from build123d import *
from OCP.BRepFilletAPI import BRepFilletAPI_MakeChamfer

# Parameters (mm, degrees)
SKETCH1_W           = 1.85
SKETCH1_H           = 38.85
SKETCH1_H_2         = 6.15
SKETCH1_W_2         = 44.85
SKETCH1_H_3         = 1.85
SKETCH1_W_3         = 0.15
BOSS_EXTRUDE1_DEPTH = 3
SKETCH1_4_W         = 120
SKETCH1_4_H         = 30
SKETCH1_4_W_2       = 30
SKETCH1_4_H_2       = 120
BOSS_EXTRUDE3_DEPTH = 4
BOSS_EXTRUDE9_DEPTH = 3
CHAMFER1_SIZE       = 2.5
CHAMFER1_SIZE2      = 9.330127019
SKETCH4_W           = 8.5
SKETCH4_H           = 30
SKETCH4_W_2         = 30
SKETCH4_H_2         = 8.5
CUT_EXTRUDE1_DEPTH  = 1.5
BOSS_EXTRUDE7_DEPTH = 4.7625
SKETCH10_R          = 14.258178215
CUT_EXTRUDE2_DEPTH  = 91.287114527
FILLET1_R           = 1.75
BOSS_EXTRUDE8_DEPTH = 4.7625
CUT_EXTRUDE3_DEPTH  = 97.69049149


with BuildPart() as part:
    # Sketch1 → Boss-Extrude1 (new body)
    with BuildSketch(Plane(origin=(0, 0, 0), x_dir=(-1, 0, 0), z_dir=(0, 0, -1))):
        with Locations((14.075, 40.575)):
            Rectangle(SKETCH1_W, SKETCH1_H)
        with Locations((14.075, 18.075)):
            Rectangle(SKETCH1_W, SKETCH1_H_2)
        with Locations((37.575, 14.075)):
            Rectangle(SKETCH1_W_2, SKETCH1_H_3)
        with Locations((14.075, 14.075)):
            Rectangle(SKETCH1_W, SKETCH1_H_3)
        with Locations((14.075, -14.075)):
            Rectangle(SKETCH1_W, SKETCH1_H_3)
        with Locations((14.075, -18.075)):
            Rectangle(SKETCH1_W, SKETCH1_H_2)
        with Locations((37.575, -14.075)):
            Rectangle(SKETCH1_W_2, SKETCH1_H_3)
        with Locations((14.075, -40.575)):
            Rectangle(SKETCH1_W, SKETCH1_H)
        with Locations((-14.075, -14.075)):
            Rectangle(SKETCH1_W, SKETCH1_H_3)
        with Locations((-14.075, -18.075)):
            Rectangle(SKETCH1_W, SKETCH1_H_2)
        with Locations((-37.575, -14.075)):
            Rectangle(SKETCH1_W_2, SKETCH1_H_3)
        with Locations((-15.075, -14.075)):
            Rectangle(SKETCH1_W_3, SKETCH1_H_3)
        with Locations((15.075, -14.075)):
            Rectangle(SKETCH1_W_3, SKETCH1_H_3)
        with Locations((15.075, 14.075)):
            Rectangle(SKETCH1_W_3, SKETCH1_H_3)
        with Locations((-37.575, 14.075)):
            Rectangle(SKETCH1_W_2, SKETCH1_H_3)
        with Locations((-15.075, 14.075)):
            Rectangle(SKETCH1_W_3, SKETCH1_H_3)
        with Locations((-14.075, 18.075)):
            Rectangle(SKETCH1_W, SKETCH1_H_2)
        with Locations((-14.075, 14.075)):
            Rectangle(SKETCH1_W, SKETCH1_H_3)
        with Locations((-14.075, 40.575)):
            Rectangle(SKETCH1_W, SKETCH1_H)
        with Locations((-14.075, -40.575)):
            Rectangle(SKETCH1_W, SKETCH1_H)
    extrude(amount=-BOSS_EXTRUDE1_DEPTH)

    # Sketch1<4> → Boss-Extrude3 (add)
    with BuildSketch(Plane(origin=(0, 0, 0), x_dir=(-1, 0, 0), z_dir=(0, 0, -1))):
        Rectangle(SKETCH1_4_W, SKETCH1_4_H)
        Rectangle(SKETCH1_4_W_2, SKETCH1_4_H_2)
    extrude(amount=BOSS_EXTRUDE3_DEPTH)

    # Sketch13 → Boss-Extrude9 (add)
    with BuildSketch(Plane.XY):
        Polygon((-12.2, 12.2), (-60, 12.2), (-60, 13.15), (-13.15, 13.15), (-13.15, 60), (-12.2, 60), align=None)
        Polygon((-60, -12.2), (-12.2, -12.2), (-12.2, -60), (-13.15, -60), (-13.15, -13.15), (-60, -13.15), align=None)
        Polygon((12.2, -60), (12.2, -12.2), (60, -12.2), (60, -13.15), (13.15, -13.15), (13.15, -60), align=None)
        Polygon((60, 12.2), (12.2, 12.2), (12.2, 60), (13.15, 60), (13.15, 13.15), (60, 13.15), align=None)
    extrude(amount=BOSS_EXTRUDE9_DEPTH)

    # Chamfer1: one chamfer whose edges measure the first distance from different faces: ONE call of the kernel's chamfer builder (chamfer() names one face for all edges)
    chamfer1_edges_1 = [part.edges().sort_by_distance(p)[0] for p in [
        (60, 0, -4),
    ]]
    chamfer1_side_1 = [part.faces().sort_by_distance(p)[0] for p in [
        (60, 0, -1.570175439),
    ]]
    chamfer1_edges_2 = [part.edges().sort_by_distance(p)[0] for p in [
        (0, 60, -4),
    ]]
    chamfer1_side_2 = [part.faces().sort_by_distance(p)[0] for p in [
        (0, 60, -1.570175439),
    ]]
    chamfer1_edges_3 = [part.edges().sort_by_distance(p)[0] for p in [
        (0, -60, -4),
    ]]
    chamfer1_side_3 = [part.faces().sort_by_distance(p)[0] for p in [
        (0, -60, -1.570175439),
    ]]
    chamfer1_edges_4 = [part.edges().sort_by_distance(p)[0] for p in [
        (-60, 0, -4),
    ]]
    chamfer1_side_4 = [part.faces().sort_by_distance(p)[0] for p in [
        (-60, 0, -1.570175439),
    ]]
    chamfer1 = BRepFilletAPI_MakeChamfer(part.part.solid().wrapped)
    for e in chamfer1_edges_1:
        chamfer1.Add(CHAMFER1_SIZE, CHAMFER1_SIZE2, e.wrapped, chamfer1_side_1[0].wrapped)  # the first distance lies on this face
    for e in chamfer1_edges_2:
        chamfer1.Add(CHAMFER1_SIZE, CHAMFER1_SIZE2, e.wrapped, chamfer1_side_2[0].wrapped)  # the first distance lies on this face
    for e in chamfer1_edges_3:
        chamfer1.Add(CHAMFER1_SIZE, CHAMFER1_SIZE2, e.wrapped, chamfer1_side_3[0].wrapped)  # the first distance lies on this face
    for e in chamfer1_edges_4:
        chamfer1.Add(CHAMFER1_SIZE, CHAMFER1_SIZE2, e.wrapped, chamfer1_side_4[0].wrapped)  # the first distance lies on this face
    add(Compound.cast(chamfer1.Shape()), mode=Mode.REPLACE)

    # Sketch4 → Cut-Extrude1 (cut)
    with BuildSketch(Plane(origin=(0, 0, -4), x_dir=(-1, 0, 0), z_dir=(0, 0, -1))):
        with Locations((-41.419872981, 0)):
            Rectangle(SKETCH4_W, SKETCH4_H)
        with Locations((-29.919872981, 0)):
            Rectangle(SKETCH4_W, SKETCH4_H)
        with Locations((0, 41.419872981)):
            Rectangle(SKETCH4_W_2, SKETCH4_H_2)
        with Locations((0, 29.919872981)):
            Rectangle(SKETCH4_W_2, SKETCH4_H_2)
        with Locations((29.919872981, 0)):
            Rectangle(SKETCH4_W, SKETCH4_H)
        with Locations((41.419872981, 0)):
            Rectangle(SKETCH4_W, SKETCH4_H)
        with Locations((0, -29.919872981)):
            Rectangle(SKETCH4_W_2, SKETCH4_H_2)
        with Locations((0, -41.419872981)):
            Rectangle(SKETCH4_W_2, SKETCH4_H_2)
    extrude(amount=-CUT_EXTRUDE1_DEPTH, mode=Mode.SUBTRACT)

    # Sketch9 → Boss-Extrude7 (add)
    with BuildSketch(Plane(origin=(-2.248627702, 2.248627702, 3.180039793), x_dir=(-0.86602540378444, -0.28867513459481, -0.40824829046386224), z_dir=(0.4999999999999977, -0.49999999999999806, -0.7071067811865507))):
        with BuildLine():
            Line((26.502649854, 26.860285477), (21.488288715, 19.768907948))
            Line((21.488288715, 19.768907948), (7.054531985, -0.643506575))
            Line((7.054531985, -0.643506575), (-2.958214479, 6.436574348))
            Line((-2.958214479, 6.436574348), (11.475542251, 26.848988872))
            Line((11.475542251, 26.848988872), (16.48990339, 33.940366401))
            ThreePointArc((16.48990339, 33.940366401), (25.036317083, 35.406699171), (26.502649854, 26.860285477))
        make_face()
        with BuildLine():
            ThreePointArc((19.161917241, 33.60764173), (16.307451178, 27.650713492), (22.309959452, 24.893384176))
            ThreePointArc((22.309959452, 24.893384176), (25.022858564, 30.799171082), (19.161917241, 33.60764173))
        make_face(mode=Mode.SUBTRACT)
    extrude(amount=BOSS_EXTRUDE7_DEPTH)

    # Sketch10 → Cut-Extrude2 (cut, through all)
    with BuildSketch(Plane.XY):
        Circle(SKETCH10_R)
    extrude(amount=CUT_EXTRUDE2_DEPTH, mode=Mode.SUBTRACT)

    # Fillet1
    fillet1_edges = [part.edges().sort_by_distance(p)[0] for p in [
        (-2.56318253, 2.56318253, -4),
        (-7.32568253, 7.32568253, -4),
        (-9.280078929, 0.60878613, -4),
        (-0.60878613, 9.280078929, -4),
    ]]
    fillet(fillet1_edges, radius=FILLET1_R)

    # Sketch11 → Boss-Extrude8 (add)
    with BuildSketch(Plane(origin=(-2.248627702, 2.248627702, 3.180039793), x_dir=(0.86602540378444, 0.28867513459481003, 0.4082482904638624), z_dir=(-0.4999999999999978, 0.4999999999999982, 0.7071067811865503))):
        with BuildLine():
            ThreePointArc((-26.502649854, 26.860285477), (-25.036317083, 35.406699171), (-16.48990339, 33.940366401))
            Line((-16.48990339, 33.940366401), (-7.126405249, 20.698380338))
            ThreePointArc((-7.126405249, 20.698380338), (-10.454022038, 27.858169656), (-11.039574704, 35.731716801))
            ThreePointArc((-11.039574704, 35.731716801), (-12.744347828, 41.802023869), (-18.161788795, 45.027890059))
            ThreePointArc((-18.161788795, 45.027890059), (-29.902759178, 42.288887582), (-36.398772273, 32.132395373))
            ThreePointArc((-36.398772273, 32.132395373), (-35.163210117, 25.949494318), (-30.008327436, 22.318783113))
            ThreePointArc((-30.008327436, 22.318783113), (-22.780260221, 19.142203051), (-17.139151713, 13.618299415))
            Line((-17.139151713, 13.618299415), (-26.502649854, 26.860285477))
        make_face()
    extrude(amount=-BOSS_EXTRUDE8_DEPTH)

    # Sketch12 → Cut-Extrude3 (cut, through all)
    with BuildSketch(Plane(origin=(-2.248627702, 2.248627702, 3.180039793), x_dir=(0.86602540378444, 0.28867513459481003, 0.4082482904638624), z_dir=(-0.4999999999999978, 0.4999999999999982, 0.7071067811865503))):
        Polygon((-25.756076527, 43.091629588), (-27.225983794, 42.459670234), (-25.971939452, 39.542823), (-24.502032185, 40.174782353), align=None)
        Polygon((-28.527874077, 41.730147071), (-26.694786972, 39.137770427), (-28.001181502, 38.214009996), (-29.834268606, 40.80638664), align=None)
        Polygon((-22.761781271, 43.84707133), (-24.330959276, 43.53453271), (-23.710765452, 40.420695106), (-22.141587447, 40.733233726), align=None)
        Polygon((-19.675853381, 43.963455868), (-21.275721515, 43.983997418), (-21.316483655, 40.809259091), (-19.716615522, 40.78871754), align=None)
        Polygon((-16.633162714, 43.435696639), (-18.193799062, 43.788420596), (-18.893735665, 40.691532844), (-17.333099317, 40.338808886), align=None)
        Polygon((-13.766689451, 42.286859254), (-15.219886716, 42.956349889), (-16.548407194, 40.072661566), (-15.095209929, 39.403170932), align=None)
        Polygon((-30.956033068, 39.822127099), (-32.04181915, 38.646938354), (-29.709803985, 36.492331599), (-28.624017903, 37.667520343), align=None)
        Polygon((-32.934431301, 37.450959299), (-33.752154873, 36.075703628), (-31.023131901, 34.453033416), (-30.205408329, 35.828289087), align=None)
        Polygon((-34.376603279, 34.720275083), (-34.890525897, 33.205057758), (-31.883766517, 32.185242563), (-31.3698439, 33.700459888), align=None)
        Polygon((-35.219519168, 31.749418455), (-35.407179947, 30.160461743), (-32.254093972, 29.788072384), (-32.066433193, 31.377029095), align=None)
        Polygon((-35.426339496, 28.668230104), (-35.279536761, 27.074979039), (-32.117929178, 27.366290716), (-32.264731914, 28.959541782), align=None)
    extrude(amount=-CUT_EXTRUDE3_DEPTH, mode=Mode.SUBTRACT)


solid = part.part
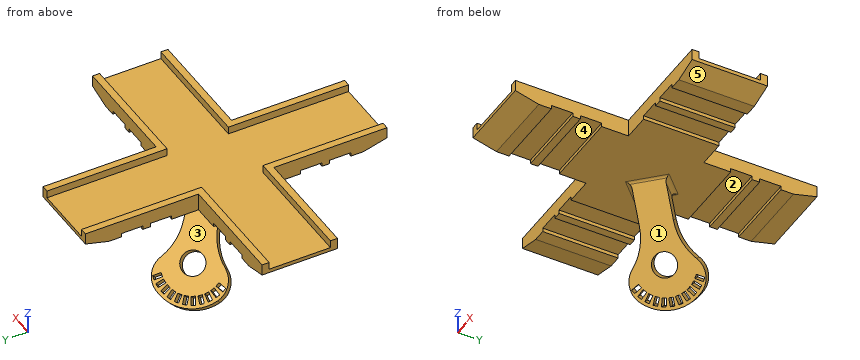
Could you check a few things on this model? Use its own coordinates, in mm. Face numbers are marked on the shaded views. A direction names the side the tool comes from. Coordinates: 2 decimals unless noted, no trailing zeros. Loops run counter-clockwise (first coordinate to the right, second up) from the corner with the lowest first, then second, coordinate; pieces in that order, holes last.
1. For the marked faces 4 and 5, which set-ups out of +Z, -Z, +X, -X, +Y, -Y let a thin tool reach every point of the face, with its end or its side?
2. I need wall thicknesses on L1, parallel to X at y = -17.5, z = -2; L2, parallel to Z at x = 46.5, y = 9. Which ranges of each line are inside material? Lowest first, please.
3. We'd pull the mould along Y, two halves only. Please class the marked faces 1, 2 and 3: released by +Y, released by -Y, zero draft, split by the parting line, or undercut.
4. For P1, Ø2.5, axis at y = -24.5, z = 2, coming from the -X side; P2, Ø12, axis at x = 32, z = -15, coming from the -Y side; P3, Ø2, axis at y = 37, z = 0.5, coming from the +X side; P4, Ø9.5, axis at x = 29, y = -1, coming from the -Z side, each with a flat end and sliding along its axis, tell me the tip position at first contact or that it passes through.
5. Imagine slicing it at A-A (y = 41). Please give me the cut outline in (x, z), and give its area (3 significant figures).
6. Imagine slicing it at C-C (z = -10). Please give me the cut outline in (x, y), and give its area (3 significant figures).
Computed values:
1. face 4: -Z, +X, -X
1. face 5: -Z, +X, +Y, -Y
2. L1: x = -15 to 15
2. L2: z = -4 to 0
3. face 1: released by -Y
3. face 2: undercut
3. face 3: released by +Y
4. P1: stops at x = -15
4. P2: passes through
4. P3: stops at x = 15
4. P4: stops at z = -4
5. outline: (-15, -2.5) - (15, -2.5) - (15, 3) - (12.2, 3) - (12.2, 0) - (-12.2, 0) - (-12.2, 3) - (-15, 3) - close
5. area: 91.8 mm2
6. outline: (-15.9, 7.23) - (-11.14, 2.47) - (-2.47, 11.14) - (-7.23, 15.9) - close
6. area: 82.6 mm2
